Check sheet for the modelled part. Datum: model origin and axes. Units: mm. Face numbers are marked on the shaded views. A direction names the side the tool comes from. Round coordinates to 2 decimals unless told otherwise and drop trailing zeros. Write each loop counter-clockwise with the first axis right and the second up, starting at its lowest first coordinate (ties: lowest second). Pieces come first, ordered by that corner, then holes. Notation, with made-up numbers: (-12.75, 82.25) - (-4.75, 82.25) arc R10 cw to (-4.75, 86.25) - close; hole circle Ø6 at (-29.75, -40). An arc over 180 degrees is marked (long way). Answer as a JSON object with one key per item and string values. Group by question number.
Item 1: Gauge pin test, flat ends, axial feed: P1, Ø1.5, axis at y = 38, z = 8, coming from the +X side; P2, Ø1.8, axis at x = 47.25, y = 4.1, coming from the -Z side; P3, Ø11, axis at x = 0, y = 23, coming from the +Z side; P4, Ø3, axis at x = -47.25, y = 4.1, coming from the -Z side. Record the tip position at first contact, or that the pin passes through.
Item 2: Release check for a two-part mould opening along X. For the marked faces 3, 4 and 5 record: pulls with the +X half, pulls with the -X half, needs draft (parallel to the pull), parting line crosses it, or undercut.
Item 3: Sectioned sample at B-B on x = 36. Record the boundary of the cut face in (y, z), plus the area to 3 significant figures.
Item 4: Sectioned sample at D-D on x = -5. Record the boundary of the cut face in (y, z).
Item 5: Sectioned sample at A-A on y = 47.9. Record the boundary of the cut face in (x, z).
Item 6: Thickness scan on line 1 (Y direction, x = 0, z = 3.25); line 2 (Y direction, x = 47.25, z = 8.8); line 3 (Z direction, x = -25, y = 17). Record the ranges inside material, lowest first.
Item 7: Sectioned sample at C-C on y = 26. Record the boundary of the cut face in (x, z), plus the area to 3 significant figures.
Item 8: Set-up check for the marked faces 1 and 2: record each of +Z, -Z, +X, -X, +Y, -Y from which the full face is reachable in a straight line by a thin tool's end or side.
```python
from build123d import *

# Parameters (mm, degrees)
BOSS_EXTRUDE1_DEPTH = 52
SKETCH2_R           = 1
CUT_EXTRUDE1_DEPTH  = 11
SKETCH3_R           = 2
CUT_EXTRUDE2_DEPTH  = 5


with BuildPart() as part:
    # Sketch1 → Boss-Extrude1 (new body)
    with BuildSketch(Plane(origin=(0, 0, 0), x_dir=(1, 0, 0), z_dir=(0, 1, 0))):
        Polygon((0, 0), (0, -4), (11.050252532, -4), (17.050252532, -10), (51.5, -10), (51.5, -7.5), (43.5, -7.5), (18.5, -6.5), (12, 0), align=None)
    extrude(amount=BOSS_EXTRUDE1_DEPTH)

    # Sketch2 → Cut-Extrude1 (cut, through all)
    with BuildSketch(Plane.XY.offset(10)):
        with Locations((47.25, 47.9)):
            Circle(SKETCH2_R)
        with Locations((47.25, 4.1)):
            Circle(SKETCH2_R)
        with BuildLine():
            Line((45.75, 52), (0, 52))
            Line((0, 52), (0, 40))
            Line((0, 40), (9.006487072, 40))
            ThreePointArc((9.006487072, 40), (10.647005463, 40.135482809), (12.243071445, 40.538260118))
            Line((12.243071445, 40.538260118), (45.75, 52))
        make_face()
        with BuildLine():
            Line((49.597069908, 44.538264905), (29.77543925, 30.69935389))
            ThreePointArc((29.77543925, 30.69935389), (25.619228249, 20.960406025), (32.541456651, 12.947669329))
            Line((32.541456651, 12.947669329), (48.463002773, 8.016455575))
            ThreePointArc((48.463002773, 8.016455575), (51.303854207, 3.486594693), (47.25, 0))
            Line((47.25, 0), (51.5, 0))
            Line((51.5, 0), (51.5, 52))
            Line((51.5, 52), (47.25, 52))
            ThreePointArc((47.25, 52), (51.161081301, 49.130220734), (49.597069908, 44.538264905))
        make_face()
    extrude(amount=-CUT_EXTRUDE1_DEPTH, mode=Mode.SUBTRACT)

    # Mirror1: part across plane


with BuildPart() as part_1:
    add(part.part)
    add(part.part.mirror(Plane(origin=(0, 52, 0), x_dir=(0, 0, 1), z_dir=(1, 0, 0))))

    # Sketch3 → Cut-Extrude2 (cut, through all)
    with BuildSketch(Plane.XY.offset(4)):
        with Locations((0, 5)):
            Circle(SKETCH3_R)
        with Locations((0, 25)):
            Circle(SKETCH3_R)
    extrude(amount=-CUT_EXTRUDE2_DEPTH, mode=Mode.SUBTRACT)


solid = part_1.part
```
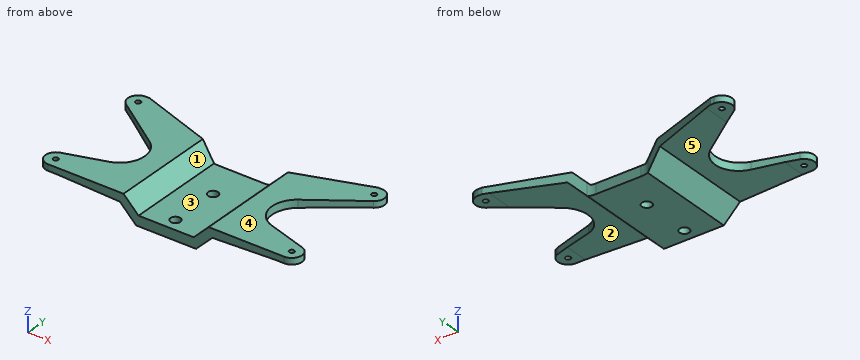
Completed:
{
 "1": {"P1": "x = 41.31", "P2": "through", "P3": "z = 4", "P4": "z = 7.5"},
 "2": {"face 3": "undercut", "face 4": "needs draft", "face 5": "pulls with the -X half"},
 "3": {"outline": "(0, 7.2) - (11.88, 7.2) - (11.88, 10) - (0, 10) - close; (35.05, 7.2) - (48.66, 7.2) - (48.66, 10) - (35.05, 10) - close", "area": "71.4 mm²"},
 "4": {"outline": "(0, 0) - (40, 0) - (40, 4) - (0, 4) - close"},
 "5": {"outline": "(-51.35, 7.5) - (-48.25, 7.5) - (-48.25, 10) - (-51.35, 10) - close; (-46.25, 7.5) - (-43.5, 7.5) - (-33.76, 7.11) - (-33.76, 10) - (-46.25, 10) - close; (33.76, 7.11) - (43.5, 7.5) - (46.25, 7.5) - (46.25, 10) - (33.76, 10) - close; (48.25, 7.5) - (51.35, 7.5) - (51.35, 10) - (48.25, 10) - close"},
 "6": {"line 1": "0 to 3, 7 to 23, 27 to 40", "line 2": "0 to 3.1, 5.1 to 8.39, 42.9 to 46.9, 48.9 to 52", "line 3": "6.76 to 10"},
 "7": {"outline": "(-26.13, 6.81) - (-18.5, 6.5) - (-12, 0) - (-1.73, 0) - (-1.73, 4) - (-11.05, 4) - (-17.05, 10) - (-26.13, 10) - close; (1.73, 0) - (12, 0) - (18.5, 6.5) - (26.13, 6.81) - (26.13, 10) - (17.05, 10) - (11.05, 4) - (1.73, 4) - close", "area": "196 mm²"},
 "8": {"face 1": "+Z, +Y, -Y", "face 2": "-Z, +X, +Y, -Y"}
}
